from build123d import *

# Parameters (mm, degrees)
SKETCH2_R          = 2.5
CUT_EXTRUDE1_DEPTH = 23


with BuildPart() as part:
    # Sketch1 → Revolve1 (revolve)
    with BuildSketch(Plane.XY, mode=Mode.PRIVATE) as revolve1_sk:
        Polygon((-8, 4.214497041), (-32.5, 4.214497041), (-32.5, -9.785502959), (-17.5, -9.785502959), (-17.5, -3.785502959), (-8, -3.785502959), align=None)
    revolve(revolve1_sk.sketch.rotate(Axis((0, 16.708579882, 0), (0, -1, 0)), 270), axis=Axis((0, 16.708579882, 0), (0, -1, 0)))

    # Sketch2 → Cut-Extrude1 (cut)
    with BuildSketch(Plane.XZ.offset(9.785502959)):
        with Locations(Location((0, 25, 0), (0, 0, 270))):
            Circle(SKETCH2_R)
        with Locations(Location((21.650635095, 12.5, 0), (0, 0, 270))):
            Circle(SKETCH2_R)
        with Locations(Location((21.650635095, -12.5, 0), (0, 0, 270))):
            Circle(SKETCH2_R)
        with Locations(Location((0, -25, 0), (0, 0, 270))):
            Circle(SKETCH2_R)
        with Locations(Location((-21.650635095, -12.5, 0), (0, 0, 270))):
            Circle(SKETCH2_R)
        with Locations(Location((-21.650635095, 12.5, 0), (0, 0, 270))):
            Circle(SKETCH2_R)
    extrude(amount=-CUT_EXTRUDE1_DEPTH, mode=Mode.SUBTRACT)


solid = part.part
The model under review builds one solid part; all positions refer to its coordinate system, in mm. A direction names the side the tool comes from. Give positions to 0.01 mm unless a question says otherwise; leave off trailing zeros. Order: outer loops, then holes, each group sorted by start corner. A loop starts at its lowest first (then second) coordinate and runs counter-clockwise, first axis right, second up. Notation, with made-up numbers: (27, 80.25) -> (83, 80.25) arc R20 ccw to (83, 89.25) -> close; hole circle Ø11 at (79.25, 66). An arc over 180 degrees is marked (long way). Write item = value, one per line. Start each with the question number.
(1) Take a section at A-A (z = 0). Write out the cut boundary in (x, y).
(2) Take a section at B-B (x = 0). Write out the cut boundary in (y, z), plus the area to 3 significant figures.
(3) For L1, parallel to Z at x = 22.5, y = -0.5; L2, parallel to X at y = -2.5, z = 12.5; L3, parallel to Z at x = 22, y = 0.5, list the stretches that pass through material, from the lowest coordinate up. Write a range as from..to.
(4) Take a section at C-C (z = -11). Write out the cut boundary in (x, y), plus the area to 3 significant figures.
(5) Tool access review of faces 5 (the cylindrical face through (-23.172, -2.884, 14.484)), 6 (the flat face through (8, -3.786, 4)): name each direction out of +Z, -Z, +X, -X, +Y, -Y from which nothing blocks a thin tool from reaching the whole face with its end or side.
(6) For pin 1 Ø6.5 at (x, z) = (-21.65, 12.5) entering from +Y; pin 2 Ø3 at (y, z) = (-4, 3) entering from -X; pin 3 Ø1 at (y, z) = (0.5, -17) entering from -X; pin 4 Ø2 at (x, y) = (-1.5, -3) entering from -Z, all flat-tipped, find the tip position at first contact; note any pin that passes through.
(7) Draft analysis for pull direction Z (two halves, no side actions). For faces 1 (the cylindrical face through (-9.76, -2.88, 31)), 2 (the cylindrical face through (0.1, -2.9, -22.5)), 3 (the flat face through (14, -9.786, 14)), 4 (the cylindrical face through (24.13, -2.88, 12.83)), state which applies: +Z half, -Z half, draft (parallel to the pull), parting line (faces both ways), or undercut.
(8) Take a section at D-D (y = -7). Write out the cut boundary in (x, z).
Returned:
q1.outline = (-32.5, -9.79) -> (-17.5, -9.79) -> (-17.5, -3.79) -> (-8, -3.79) -> (-8, 4.21) -> (-32.5, 4.21) -> close; (8, -3.79) -> (17.5, -3.79) -> (17.5, -9.79) -> (32.5, -9.79) -> (32.5, 4.21) -> (8, 4.21) -> close
q2.outline = (-9.79, -32.5) -> (4.21, -32.5) -> (4.21, -27.5) -> (-9.79, -27.5) -> close; (-9.79, -22.5) -> (4.21, -22.5) -> (4.21, -8) -> (-3.79, -8) -> (-3.79, -17.5) -> (-9.79, -17.5) -> close; (-9.79, 17.5) -> (-3.79, 17.5) -> (-3.79, 8) -> (4.21, 8) -> (4.21, 22.5) -> (-9.79, 22.5) -> close; (-9.79, 27.5) -> (4.21, 27.5) -> (4.21, 32.5) -> (-9.79, 32.5) -> close
q2.area = 432 mm²
q3.L1 = -23.45..-14.85, -10.15..10.15, 14.85..23.45
q3.L2 = -30..-24.15, -19.15..19.15, 24.15..30
q3.L3 = -23.92..-14.98, -10.02..10.02, 14.98..23.92
q4.outline = (-30.58, -9.79) -> (-23.65, -9.79) -> (-23.65, 4.21) -> (-30.58, 4.21) -> close; (-19.65, -9.79) -> (-13.61, -9.79) -> (-13.61, -3.79) -> (13.61, -3.79) -> (13.61, -9.79) -> (19.65, -9.79) -> (19.65, 4.21) -> (-19.65, 4.21) -> close; (23.65, -9.79) -> (30.58, -9.79) -> (30.58, 4.21) -> (23.65, 4.21) -> close
q4.area = 581 mm²
q5.face_5 = +Y, -Y
q5.face_6 = -Y
q6.pin_1 = 4.21
q6.pin_2 = -32.47
q6.pin_3 = -28
q6.pin_4 = -32.5
q7.face_1 = parting line
q7.face_2 = undercut
q7.face_3 = draft
q7.face_4 = undercut
q8.outline = circle Ø65 at (0, 0); hole circle Ø5 at (-21.65, -12.5); hole circle Ø5 at (-21.65, 12.5); hole circle Ø35 at (0, 0); hole circle Ø5 at (0, -25); hole circle Ø5 at (0, 25); hole circle Ø5 at (21.65, -12.5); hole circle Ø5 at (21.65, 12.5)
